Autodesk Fusion 360 part; units mm, degrees
sketch "Sketch1" plane through (0, 0, 0) normal (1, 0, 0) x (0, 1, 0)
  line L0 (0, 0) -> (22.5, 0)
  line L1 (22.5, 0) -> (22.5, 33.4)
  line L2 (22.5, 33.4) -> (0, 33.4)
  line L3 (0, 33.4) -> (0, 29.4)
  line L4 (0, 29.4) -> (2.5, 29.4)
  line L5 (0, 0) -> (0, 4)
  line L6 (0, 4) -> (2.5, 4)
  line L7 (2.5, 29.4) -> (2.5, 4)
  line L8 (2.5, 29.4) -> (2.5, 33.4) construction
  line L9 (0, 29.4) -> (0, 4)
  dimension "d1" = 25.4
  dimension "d4" = 4
  dimension "d5" = 2.5
  dimension "d6" = 20
extrude "Extrude1" add sketch "Sketch1" along normal blind 20 contours L0 L1 L2 L3 L4 L5 L6 L7
extrude "Extrude2" add sketch "Sketch1" against normal blind 4
sketch "Sketch2" plane through (0, 2.5, 0) normal (0, -1, 0) x (1, 0, 0)
  line L0 (0, 29.4) -> (0, 4)
  line L1 (0, 4) -> (20, 4)
  line L2 (20, 4) -> (20, 29.4)
  line L3 (20, 29.4) -> (0, 29.4)
  circle A0 centre (10, 16.7) radius 2
  line L4 (10, 16.7) -> (10, 29.4) construction
  line L5 (10, 16.7) -> (0, 16.7) construction
  dimension "d11" = 4
extrude "Extrude3" cut sketch "Sketch2" against normal up to surface (20 mm away) contours A0
chamfer "Chamfer1" distance 4 angle 45 1 edges at (8.1353, 2.5, 17.4232)
equation "d1 = 1\""
Model file for the job. Use its own axes, mm. A direction names the side the tool comes from. Give positions to 0.01 mm unless a question says otherwise; leave off trailing zeros. Write each loop counter-clockwise with the first axis right and the second up, starting at its lowest first coordinate (ties: lowest second). Pieces come first, ordered by that corner, then holes. Notation, with made-up numbers: (-1.5, 18) - (42.5, 18) arc R14 cw to (42.5, 40) - close; hole circle Ø10 at (28, 11.25). An arc over 180 degrees is marked (long way). One line per question, with ' | ' between items. Start each with the question number.
(1) Pin check, flat tips, straight feed: P1, Ø12, axis at x = 3, z = 9.5, coming from the -Y side; P2, Ø6, axis at x = 11, z = 16, coming from the -Y side; P3, Ø2, axis at y = 1, z = 22, coming from the +X side; P4, Ø3, axis at x = 13, z = 7, coming from the -Y side. Stop position of each tip, or through.
(2) Slice it at D-D on x = 2.5. Write the cut outline in (y, z), plus the area to 3 significant figures.
(3) Slice it at A-A on z = 16.7. Write the cut outline in (x, y).
(4) Wall check: line 1 along Z through (x, y) = (10, 12); line 2 along Y through (x, z) = (11.75, 6); line 3 along Z through (x, y) = (8.75, 3). Give the ranges that are in metal, low to high. Write a range as from..to.
(5) Two-plate mould, pull along X, no slides. Class faces 3 (the face through (-4, 11, 17)), 4 (the face through (9.566, 14.388, 14.748)), 5 (the face through (9.71, 6.25, 18.93)), 6 (the face through (0, 1, 17)): +X half, -X half, draft (parallel to the pull), parting line (faces both ways), or undercut.
(6) Slice it at C-C on x = 10. Write the cut outline in (y, z), plus the area to 3 significant figures.
(7) Slice it at B-B on y = 9.75. Write the cut outline in (x, z).
(8) 3-axis set-ups, long thin cutter, end or side, ignore diameter. For faces 1 (the face through (8, 11, 0)), 2 (the face through (10, 1, 29.4)): which of +Z, -Z, +X, -X, +Y, -Y reach the whole face in a straight line?
Results below:
1) P1: y = 0 | P2: y = 4.28 | P3: x = 0 | P4: y = 2.5
2) outline: (0, 0) - (22.5, 0) - (22.5, 33.4) - (0, 33.4) - (0, 29.4) - (2.5, 29.4) - (2.5, 4) - (0, 4) - close | area: 688 mm^2
3) outline: (-4, 0) - (0, 0) - (0, 2.5) - (4, 2.5) - (8, 6.5) - (8, 22.5) - (-4, 22.5) - close; (12, 6.5) - (16, 2.5) - (20, 2.5) - (20, 22.5) - (12, 22.5) - close
4) line 1: 0..14.7, 18.7..33.4 | line 2: 2.5..22.5 | line 3: 0..11.34, 22.06..33.4
5) face 3: -X half | face 4: undercut | face 5: undercut | face 6: +X half
6) outline: (0, 0) - (22.5, 0) - (22.5, 14.7) - (6.5, 14.7) - (2.5, 10.7) - (2.5, 4) - (0, 4) - close; (0, 29.4) - (2.5, 29.4) - (2.5, 22.7) - (6.5, 18.7) - (22.5, 18.7) - (22.5, 33.4) - (0, 33.4) - close | area: 592 mm^2
7) outline: (-4, 0) - (20, 0) - (20, 33.4) - (-4, 33.4) - close; hole circle Ø4 at (10, 16.7)
8) face 1: -Z, +X, -X, +Y, -Y | face 2: +X, -Y
